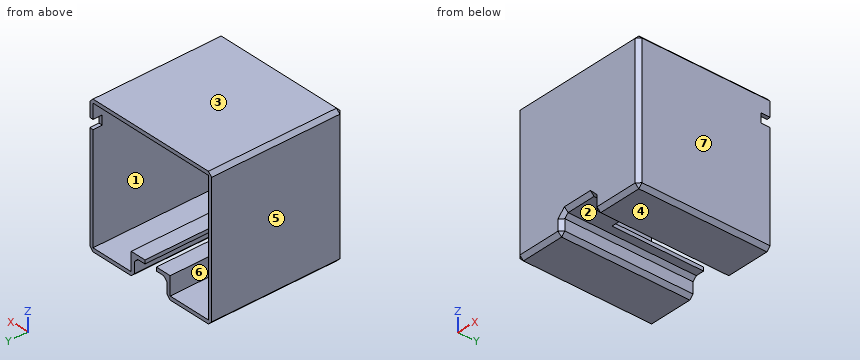
Autodesk Fusion 360 part; units mm, degrees
sketch "Sketch1" plane through (0, 0, 0) normal (0, 1, 0) x (1, 0, 0)
  line L0 (0, 0) -> (75, 0)
  line L1 (75, 0) -> (75, 75)
  line L2 (75, 75) -> (0, 75)
  line L3 (0, 75) -> (0, 0)
  dimension "d1" = 75
  dimension "d2" = 75
extrude "Extrude1" add sketch "Sketch1" along normal blind 72
sketch "Sketch2" plane through (0, 0, 0) normal (0, -1, 0) x (1, 0, 0)
  line L0 (0, 0) -> (0, -75)
  line L1 (0, -75) -> (75, -75)
  line L2 (75, -75) -> (75, 0)
  line L3 (75, 0) -> (0, 0)
  line L4 (2, -73) -> (73, -73)
  line L5 (73, -73) -> (73, -2)
  line L6 (73, -2) -> (2, -2)
  line L7 (2, -2) -> (2, -73)
  line L8 (27.5, -75) -> (27.5, -73)
  line L9 (47.5, -75) -> (47.5, -73)
  line L10 (27.5, -73) -> (27.5, -65)
  line L11 (47.5, -73) -> (47.5, -65)
  line L12 (47.5, -65) -> (27.5, -65)
  line L13 (27.5, -73) -> (25.5, -73)
  line L14 (25.5, -73) -> (25.5, -63)
  line L15 (25.5, -63) -> (49.5, -63)
  line L16 (49.5, -63) -> (49.5, -73)
  line L17 (34, -65) -> (41, -65)
  line L18 (41, -65) -> (41, -61)
  line L19 (41, -61) -> (34, -61)
  line L20 (34, -61) -> (34, -65)
  line L21 (34, -65) -> (41, -61) construction
  line L22 (41, -65) -> (34, -61) construction
  point P0 (37.5, -63)
  dimension "d7" = -2
  dimension "d9" = 24
extrude "Extrude2" cut sketch "Sketch2" against normal blind 70 from surface at -2 contours L4 L5 L6 L7 L14 L15 L16 L18 L19 L20 | L15 L18 L19 L20
extrude "Extrude3" cut sketch "Sketch2" against normal blind 72 contours L1 L4 L8 L9 | L4 L10 L11 L12 L17
extrude "Extrude4" cut sketch "Sketch2" against normal blind 50 from surface at -22 contours L12 L15 L17 L18 L20
sketch "Sketch3" plane through (75, 0, 0) normal (1, 0, 0) x (0, 1, 0)
  line L0 (0, 0) -> (0, -75)
  line L1 (0, -75) -> (72, -75)
  line L2 (72, -75) -> (72, 0)
  line L3 (72, 0) -> (0, 0)
  line L4 (67, -10) -> (72, -10)
  line L5 (72, -10) -> (72, -15)
  line L6 (72, -15) -> (67, -15)
  line L7 (67, -15) -> (67, -10)
  dimension "d18" = 5
extrude "Extrude5" cut sketch "Sketch3" against normal blind 2 contours L2 L4 L5 L6 L7
chamfer "Chamfer1" distance 2 angle 45 1 edges at (13.75, 0, -75) measured on face at (18.3333, 48, -75)
chamfer "Chamfer1" distance 2 angle 45 1 edges at (27.5, 0, -70) measured on face at (40.8333, 0, -21.6667)
chamfer "Chamfer1" distance 2 angle 45 6 edges at (37.5, 0, -65) (47.5, 0, -70) (61.25, 0, -75) (75, 0, -37.5) (0, 0, -37.5) (37.5, 0, 0) measured on face at (40.8333, 0, -21.6667) measured on face at (40.8333, 0, -21.6667) measured on face at (65.8333, 48, -75) measured on face at (75, 22.3333, -30) measured on face at (0, 24, -50) measured on face at (25, 24, 0)
chamfer "Chamfer1" distance 2 angle 45 6 edges at (75, 36, -75) (47.5, 36, -75) (27.5, 36, -75) (0, 36, -75) (75, 36, 0) (0, 36, 0) measured on face at (75, 22.3333, -30) measured on face at (65.8333, 48, -75) measured on face at (18.3333, 48, -75) measured on face at (18.3333, 48, -75) measured on face at (25, 24, 0) measured on face at (0, 24, -50)
chamfer "Chamfer1" distance 2 angle 45 2 edges at (47.5, 36, -65) (27.5, 36, -65) measured on face at (47.5, 24, -71.6667) measured on face at (38.6667, 7.3333, -65)
CAD build for the part. Positions are in the model's coordinates, mm. Face numbers are marked on the shaded views. A direction names the side the tool comes from. Coordinates: 2 decimals unless noted, no trailing zeros. Order: outer loops, then holes, each group sorted by start corner. A loop starts at its lowest first (then second) coordinate and runs counter-clockwise, first axis right, second up. Notation, with made-up numbers: (34, 48.5) -> (86, 48.5) arc R18 ccw to (86, 72.5) -> close; hole circle Ø7 at (36.25, -31). An arc over 180 degrees is marked (long way). Answer in a Markdown table with one row per item.
1) Band-saw the part on C-C (y = 18.5). List the corners of the cut face in (x, z).
Check values:
| item | result |
|---|---|
| outline | (0, -73) -> (2, -75) -> (25.5, -75) -> (27.5, -73) -> (27.5, -67) -> (29.5, -65) -> (45.5, -65) -> (47.5, -67) -> (47.5, -73) -> (49.5, -75) -> (73, -75) -> (75, -73) -> (75, -2) -> (73, 0) -> (2, 0) -> (0, -2) -> close; hole (2, -73) -> (25.5, -73) -> (25.5, -63) -> (49.5, -63) -> (49.5, -73) -> (73, -73) -> (73, -2) -> (2, -2) -> close |
2) Band-saw the part on B-B (x = 9.5). List the corners of the cut face in (y, z).
Check values:
| item | result |
|---|---|
| outline | (0, -73) -> (2, -75) -> (72, -75) -> (72, -73) -> (2, -73) -> (2, -2) -> (72, -2) -> (72, 0) -> (2, 0) -> (0, -2) -> close |
3) Band-saw the part on A-A (z = -13.5). List the corners of the cut face in (x, y).
Check values:
| item | result |
|---|---|
| outline | (0, 2) -> (2, 0) -> (73, 0) -> (75, 2) -> (75, 67) -> (73, 67) -> (73, 2) -> (2, 2) -> (2, 72) -> (0, 72) -> close |
4) Mould opens along X. For the marked faces 4, 5, 6 and 7 say: pulls with the +X half, pulls with the -X half, needs draft (parallel to the pull), parting line crosses it, or undercut.
Check values:
| item | result |
|---|---|
| face 4 | needs draft |
| face 5 | pulls with the -X half |
| face 6 | undercut |
| face 7 | pulls with the +X half |
5) Which spindle directions (+Z, -Z, +X, -X, +Y, -Y) get a long thin tool onto all of the face, cutting with end or side? Do the marked faces 1, 2 and 3. Say none if no direction does.
Check values:
| item | result |
|---|---|
| face 1 | +Y |
| face 2 | -Z, +Y, -Y |
| face 3 | +Z, +X, -X, +Y, -Y |
6) Band-saw the part on D-D (y = 31.5). List the corners of the cut face in (x, z).
Check values:
| item | result |
|---|---|
| outline | (0, -73) -> (2, -75) -> (25.5, -75) -> (27.5, -73) -> (27.5, -67) -> (29.5, -65) -> (34, -65) -> (34, -63) -> (25.5, -63) -> (25.5, -73) -> (2, -73) -> (2, -2) -> (73, -2) -> (73, -73) -> (49.5, -73) -> (49.5, -63) -> (41, -63) -> (41, -65) -> (45.5, -65) -> (47.5, -67) -> (47.5, -73) -> (49.5, -75) -> (73, -75) -> (75, -73) -> (75, -2) -> (73, 0) -> (2, 0) -> (0, -2) -> close |
7) Flat gauge pins, fed straight in: P1, Ø10, axis at x = 41.5, z = -38.5, coming from the -Y side; P2, Ø1.5, axis at x = 52.5, z = -45.5, coming from the +Y side; P3, Ø1.6, axis at x = 36.5, z = -64, coming from the +Y side; P4, Ø1.6, axis at x = 74, y = 68.5, coming from the -Z side. Where does each tip first touch, or does it go through?
Check values:
| item | result |
|---|---|
| P1 | y = 0 |
| P2 | y = 2 |
| P3 | y = 22 |
| P4 | z = -74.8 |
8) Drill centre lines: line 1 (X direction, y = 35, z = -46); line 2 (Z direction, x = 53, y = 56); line 3 (Y direction, x = 61, z = -57.5). Where is each one in solid material? Low to high.
Check values:
| item | result |
|---|---|
| line 1 | 0 to 2, 73 to 75 |
| line 2 | -75 to -73, -2 to 0 |
| line 3 | 0 to 2 |
